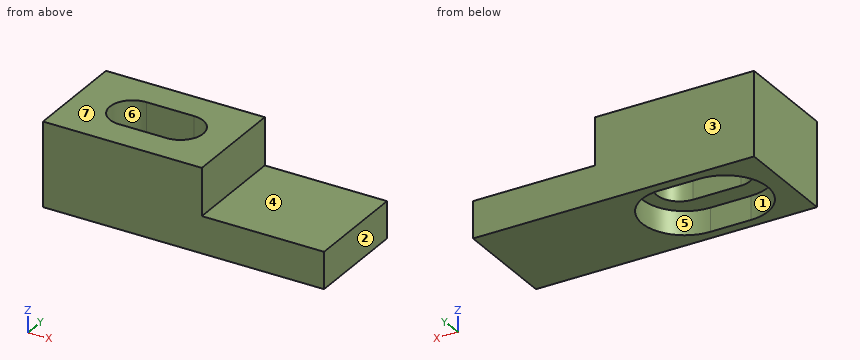
from build123d import *

# Parameters (mm, degrees)
SKETCH_W        = 23.8
SKETCH_H        = 8.85
PAD_DEPTH       = 7.1
SKETCH001_W     = 10.35
SKETCH001_H     = 8.85
POCKET_DEPTH    = 4
POCKET001_DEPTH = 7.101
POCKET002_DEPTH = 2


with BuildPart() as part:
    # Sketch → Pad (new body)
    with BuildSketch(Plane.XY):
        Rectangle(SKETCH_W, SKETCH_H)
    extrude(amount=PAD_DEPTH)

    # Sketch001 → Pocket (cut)
    with BuildSketch(Plane.XY.offset(7.1)):
        with Locations((6.725, 0)):
            Rectangle(SKETCH001_W, SKETCH001_H)
    extrude(amount=-POCKET_DEPTH, mode=Mode.SUBTRACT)

    # Sketch002 → Pocket001 (cut, through all)
    with BuildSketch(Plane.XY.offset(7.1)):
        with BuildLine():
            ThreePointArc((-6.975, 1.925), (-8.9, 0), (-6.975, -1.925))
            Line((-6.975, -1.925), (-2.925, -1.925))
            ThreePointArc((-2.925, -1.925), (-1, 0), (-2.925, 1.925))
            Line((-6.975, 1.925), (-2.925, 1.925))
        make_face()
    extrude(amount=-POCKET001_DEPTH, mode=Mode.SUBTRACT)

    # Sketch003 → Pocket002 (cut)
    with BuildSketch(Plane(origin=(0, 0, 0), x_dir=(1, 0, 0), z_dir=(0, 0, -1))):
        with BuildLine():
            ThreePointArc((-6.8, 3.6), (-10.4, 0), (-6.8, -3.6))
            Line((-6.8, -3.6), (-3.36, -3.6))
            ThreePointArc((-3.36, -3.6), (0.24, 0), (-3.36, 3.6))
            Line((-6.8, 3.6), (-3.36, 3.6))
        make_face()
    extrude(amount=-POCKET002_DEPTH, mode=Mode.SUBTRACT)


solid = part.part
CAD build for the part. Positions are in the model's coordinates, mm. Face numbers are marked on the shaded views. A direction names the side the tool comes from. Round coordinates to 2 decimals unless told otherwise and drop trailing zeros. Write each loop counter-clockwise with the first axis right and the second up, starting at its lowest first coordinate (ties: lowest second). Pieces come first, ordered by that corner, then holes. Notation, with made-up numbers: M -18.75,54.25 L 0.25,54.25 A16 ccw 0.25,66.25 Z; hole C 1.25,-3.75 d1. An arc over 180 degrees is marked long. Use a Markdown table: item, result. Add a question column.
1. 3-axis set-ups, long thin cutter, end or side, ignore diameter. For the marked faces 4, 5, 6 and 7: which of +Z, -Z, +X, -X, +Y, -Y reach the whole face in a straight line?
2. Drill centre lines: probe 1 along Y at (x, z) = (-6.5, 2.75) (3 decimals); probe 2 along Y at (x, z) = (-7, 0.75) (3 decimals); probe 3 along X at (y, z) = (3.25, 4.5). Where is each one in solid material? Low to high.
3. Slice it at A-A on x = -6.25. Give the cut face in (y, z) (3 decimals).
4. Pull direction X, two halves, no side cores. Call the marked faces 1, 2 and 3: released by +X, released by -X, zero draft, split by the parting line, or undercut.
5. Slice it at D-D on y = 4. Give the cut face in (x, z), then the cut area to 3 significant figures.
6. Flat gauge pins, fed straight in: P1, Ø4.5, axis at x = 6, y = -1.5, coming from the +Z side; P2, Ø1.2, axis at y = 0.5, z = 5.5, coming from the +X side. Where does each tip first touch, or does it go through?
7. Slice it at B-B on y = 0. Give the cut face in (x, z), then the cut area to 3 significant figures.
8. Slice it at C-C on z = 2.25. Give the cut face in (x, y) (3 decimals), then the cut area to 3 significant figures.
Reply:
| question | item | result |
|---|---|---|
| 1 | face 4 | +Z, +X, +Y, -Y |
| 1 | face 5 | -Z |
| 1 | face 6 | +Z, -Z |
| 1 | face 7 | +Z, +X, -X, +Y, -Y |
| 2 | probe 1 | y = -4.425 to -1.925, 1.925 to 4.425 |
| 2 | probe 2 | y = -4.425 to -3.594, 3.594 to 4.425 |
| 2 | probe 3 | x = -11.9 to 1.55 |
| 3 | outline | M -4.425,0 L -3.6,0 L -3.6,2 L -1.925,2 L -1.925,7.1 L -4.425,7.1 Z; M 1.925,2 L 3.6,2 L 3.6,0 L 4.425,0 L 4.425,7.1 L 1.925,7.1 Z |
| 4 | face 1 | undercut |
| 4 | face 2 | released by +X |
| 4 | face 3 | zero draft |
| 5 | outline | M -11.9,0 L 11.9,0 L 11.9,3.1 L 1.55,3.1 L 1.55,7.1 L -11.9,7.1 Z |
| 5 | area | 128 mm^2 |
| 6 | P1 | stops at z = 3.1 |
| 6 | P2 | stops at x = 1.55 |
| 7 | outline | M -11.9,0 L -10.4,0 L -10.4,2 L -8.9,2 L -8.9,7.1 L -11.9,7.1 Z; M -1,2 L 0.24,2 L 0.24,0 L 11.9,0 L 11.9,3.1 L 1.55,3.1 L 1.55,7.1 L -1,7.1 Z |
| 7 | area | 66.0 mm^2 |
| 8 | outline | M -11.9,-4.425 L 11.9,-4.425 L 11.9,4.425 L -11.9,4.425 Z; hole M -6.975,-1.925 L -2.925,-1.925 A1.925 ccw -2.925,1.925 L -6.975,1.925 A1.925 ccw Z |
| 8 | area | 183 mm^2 |
